Design review of the part built by this model. Coordinates are the model's own, in mm. Coordinates: 2 decimals unless noted, no trailing zeros. Write each loop counter-clockwise with the first axis right and the second up, starting at its lowest first coordinate (ties: lowest second). Pieces come first, ordered by that corner, then holes. Notation, with made-up numbers: (-19, -10.5) - (15, -10.5) arc R24 ccw to (15, 10.5) - close; hole circle Ø6 at (-14.5, -14). An arc over 180 degrees is marked (long way). Use a Markdown table: item, result.
from build123d import *

# Parameters (mm, degrees)
PAD_DEPTH = 10


with BuildPart() as part:
    # Sketch → Pad (new body)
    with BuildSketch(Plane.XY):
        with BuildLine():
            ThreePointArc((15.075, -26.110666), (30.15, 0), (15.075, 26.110666))
            Line((15.075, 29.028831), (15.075, 26.110666))
            Line((66.494071, 25.204654), (15.075, 29.028831))
            Line((66.494071, 25.204654), (66.494071, 20.16834))
            ThreePointArc((66.494071, 20.16834), (55.627916, 0), (66.494071, -20.16834))
            Line((66.494071, -20.16834), (66.494071, -25.204654))
            Line((15.075, -29.028831), (66.494071, -25.204654))
            Line((15.075, -26.110666), (15.075, -29.028831))
        make_face()
    extrude(amount=PAD_DEPTH)


solid = part.part
(1) Take a section at A-A on z = 3. Write out the cut boundary in (x, y) (3 decimals).
Determined:
| item | result |
|---|---|
| outline | (15.075, -29.029) - (66.494, -25.205) - (66.494, -20.168) arc R24.15 cw to (66.494, 20.168) - (66.494, 25.205) - (15.075, 29.029) - (15.075, 26.111) arc R30.15 cw to (15.075, -26.111) - close |
(2) For pin 1 (2 mm diameter, centred on y = -13.5, z = 2, fed in from -X); pin 2 (10 mm diameter, centred on x = 23.5, y = -5.5, fed in from +Z); pin 3 (5 mm diameter, centred on x = 54, z = 2, fed in from +Y); pin 4 (1.5 mm diameter, centred on y = -21, z = 7, fed in from -X), all flat-tipped, find the tip position at first contact; note any pin that passes through.
Determined:
| item | result |
|---|---|
| pin 1 | x = 26.43 |
| pin 2 | through |
| pin 3 | y = 26.32 |
| pin 4 | x = 20.88 |
(3) Take a section at C-C on y = -9. Write out the cut boundary in (x, z), and give its area (3 significant figures).
Determined:
| item | result |
|---|---|
| outline | (28.78, 0) - (57.37, 0) - (57.37, 10) - (28.78, 10) - close |
| area | 286 mm2 |
(4) Take a section at B-B on x = 20. Write out the cut boundary in (y, z), and give its area (3 significant figures).
Determined:
| item | result |
|---|---|
| outline | (-28.66, 0) - (-22.56, 0) - (-22.56, 10) - (-28.66, 10) - close; (22.56, 0) - (28.66, 0) - (28.66, 10) - (22.56, 10) - close |
| area | 122 mm2 |
(5) For L1, parallel to Y at x = 25.5, z = 6.5; L2, parallel to Y at x = 19.5, z = 6; L3, parallel to Y at x = 44.5, z = 8, list the stretches that pass through material, from the lowest coordinate up. Write a range as from..to.
Determined:
| item | result |
|---|---|
| L1 | -28.25..-16.09, 16.09..28.25 |
| L2 | -28.7..-23, 23..28.7 |
| L3 | -26.84..26.84 |
(6) Draft analysis for pull direction Y (two halves, no side actions). For faces 1 (the cylindrical face through (30.147, -0.442, 4.93)), 2 (the flat face through (41, 0, 10)), 3 (the flat face through (41.14, 27.09, 4.93)), state which applies: +Y half, -Y half, draft (parallel to the pull), parting line (faces both ways), or undercut.
Determined:
| item | result |
|---|---|
| face 1 | undercut |
| face 2 | draft |
| face 3 | +Y half |
(7) Take a section at D-D on x = 40.5. Write out the cut boundary in (y, z), and give its area (3 significant figures).
Determined:
| item | result |
|---|---|
| outline | (-27.14, 0) - (27.14, 0) - (27.14, 10) - (-27.14, 10) - close |
| area | 543 mm2 |
